Drawing for the job (mm, zero at the part's lowest x, y, z). Coordinates: 2 decimals unless noted, no trailing zeros. Write each loop counter-clockwise with the first axis right and the second up, starting at its lowest first coordinate (ties: lowest second). Pieces come first, ordered by that corner, then holes. Notation, with made-up numbers: (-35.5, 3) -> (-24.5, 3) arc R28 ccw to (-24.5, 31) -> close; hole circle Ø8 at (-34.5, 14.5). An arc over 180 degrees is marked (long way). Write item = value, one per line. Start each with the question number.
Q1. Probe line 1 (X direction, y = 0.5, z = 10); line 2 (X direction, y = 1.35, z = 30); line 3 (X direction, y = 1.6, z = 52.5). List the from-to ranges inside material, lowest first.
Q2. Band-saw the part on C-C, the plane z = 50. List the corners of the cut face in (x, y).
Q3. Band-saw the part on D-D, the plane z = 10. List the corners of the cut face in (x, y).
Q4. Pin check, flat tips, straight feed: P1, Ø4, axis at x = 13, z = 12.5, coming from the -Y side; P2, Ø1, axis at y = 1.5, z = 40, coming from the +X side; P3, Ø1, axis at x = 28.5, y = 0, coming from the +Z side. Stop position of each tip, or through.
Q5. Band-saw the part on A-A, the plane y = 1.35. List the corners of the cut face in (x, z) (1 decimal), plus the area to 3 significant figures.
Q6. Band-saw the part on B-B, the plane x = 50. List the corners of the cut face in (y, z), plus the area to 3 significant figures.
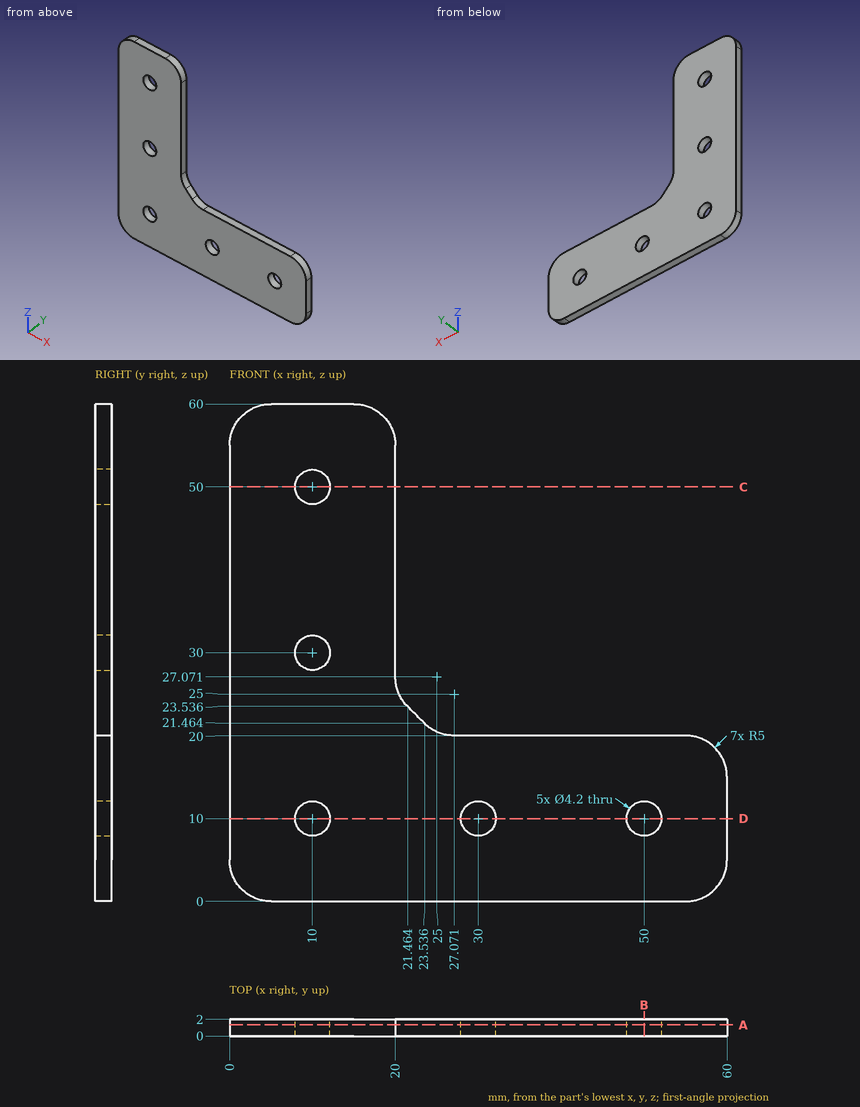
Ans:
q1.line_1 = 0 to 7.9, 12.1 to 27.9, 32.1 to 47.9, 52.1 to 60
q1.line_2 = 0 to 7.9, 12.1 to 20
q1.line_3 = 0 to 20
q2.outline = (0, 0) -> (7.9, 0) -> (7.9, 2) -> (0, 2) -> close; (12.1, 0) -> (20, 0) -> (20, 2) -> (12.1, 2) -> close
q3.outline = (0, 0) -> (7.9, 0) -> (7.9, 2) -> (0, 2) -> close; (12.1, 0) -> (27.9, 0) -> (27.9, 2) -> (12.1, 2) -> close; (32.1, 0) -> (47.9, 0) -> (47.9, 2) -> (32.1, 2) -> close; (52.1, 0) -> (60, 0) -> (60, 2) -> (52.1, 2) -> close
q4.P1 = 0
q4.P2 = 20
q4.P3 = 20
q5.outline = (0, 5) arc R5 ccw to (5, 0) -> (55, 0) arc R5 ccw to (60, 5) -> (60, 15) arc R5 ccw to (55, 20) -> (27.1, 20) arc R5 cw to (23.5, 21.5) -> (21.5, 23.5) arc R5 cw to (20, 27.1) -> (20, 55) arc R5 ccw to (15, 60) -> (5, 60) arc R5 ccw to (0, 55) -> close; hole circle Ø4.2 at (10, 10); hole circle Ø4.2 at (10, 30); hole circle Ø4.2 at (10, 50); hole circle Ø4.2 at (30, 10); hole circle Ø4.2 at (50, 10)
q5.area = 1,920 mm2
q6.outline = (0, 0) -> (2, 0) -> (2, 7.9) -> (0, 7.9) -> close; (0, 12.1) -> (2, 12.1) -> (2, 20) -> (0, 20) -> close
q6.area = 31.6 mm2
